Check sheet for the modelled part. Datum: model origin and axes. Units: mm. A direction names the side the tool comes from. Coordinates: 2 decimals unless noted, no trailing zeros. Order: outer loops, then holes, each group sorted by start corner. A loop starts at its lowest first (then second) coordinate and runs counter-clockwise, first axis right, second up. Notation, with made-up numbers: (-37.5, -8) -> (-33.5, -8) arc R35 ccw to (-33.5, 25) -> close; hole circle Ø5 at (16, 46.25). An arc over 180 degrees is marked (long way). Put each result on its own line as item: value. Start each with the question number.
```python
from build123d import *

# Parameters (mm, degrees)
BOSS_EXTRUDE1_DEPTH = 7
SKETCH2_R           = 7
SKETCH2_R_2         = 4
BOSS_EXTRUDE2_DEPTH = 5
SKETCH3_R           = 4
CUT_EXTRUDE1_DEPTH  = 15
BOSS_EXTRUDE3_DEPTH = 12
SKETCH5_R           = 1.5
CUT_EXTRUDE2_DEPTH  = 12


with BuildPart() as part:
    # Sketch1 → Boss-Extrude1 (new body)
    with BuildSketch(Plane.XY):
        with BuildLine():
            ThreePointArc((-12.439687438, -6.422941417), (-10.325628022, -6.417742109), (-8.410516827, -5.522407894))
            ThreePointArc((-8.410516827, -5.522407894), (-7.866397461, -6.273242641), (-7.255465658, -6.970796248))
            ThreePointArc((-7.255465658, -6.970796248), (-8.554504306, -8.638661002), (-9.029995733, -10.698559579))
            ThreePointArc((-9.029995733, -10.698559579), (-8.728857226, -10.945640755), (-8.42096127, -11.184248356))
            ThreePointArc((-8.42096127, -11.184248356), (-6.518515447, -10.262307937), (-5.181530838, -8.624704077))
            ThreePointArc((-5.181530838, -8.624704077), (-4.365521241, -9.065098264), (-3.512433539, -9.428498973))
            ThreePointArc((-3.512433539, -9.428498973), (-3.959167524, -11.494824938), (-3.493813999, -13.557037425))
            ThreePointArc((-3.493813999, -13.557037425), (-3.115293075, -13.648990771), (-2.734360446, -13.730377742))
            ThreePointArc((-2.734360446, -13.730377742), (-1.420330943, -12.07429782), (-0.926279119, -10.018771843))
            ThreePointArc((-0.926279119, -10.018771843), (0, -10.0615), (0.926279119, -10.018771843))
            ThreePointArc((0.926279119, -10.018771843), (1.420330943, -12.07429782), (2.734360446, -13.730377742))
            ThreePointArc((2.734360446, -13.730377742), (3.115293075, -13.648990771), (3.493813999, -13.557037425))
            ThreePointArc((3.493813999, -13.557037425), (3.959167524, -11.494824938), (3.512433539, -9.428498973))
            ThreePointArc((3.512433539, -9.428498973), (4.365521241, -9.065098264), (5.181530838, -8.624704077))
            ThreePointArc((5.181530838, -8.624704077), (6.518515447, -10.262307937), (8.42096127, -11.184248356))
            ThreePointArc((8.42096127, -11.184248356), (8.728857226, -10.945640755), (9.029995733, -10.698559579))
            ThreePointArc((9.029995733, -10.698559579), (8.554504306, -8.638661002), (7.255465658, -6.970796248))
            ThreePointArc((7.255465658, -6.970796248), (7.866397461, -6.273242641), (8.410516827, -5.522407894))
            ThreePointArc((8.410516827, -5.522407894), (10.325628022, -6.417742109), (12.439687438, -6.422941417))
            ThreePointArc((12.439687438, -6.422941417), (12.613564151, -6.074372348), (12.777676066, -5.7211008))
            ThreePointArc((12.777676066, -5.7211008), (11.455516597, -4.071504309), (9.561463821, -3.132441835))
            ThreePointArc((9.561463821, -3.132441835), (9.809237188, -2.238894377), (9.97369681, -1.3263311))
            ThreePointArc((9.97369681, -1.3263311), (12.087623332, -1.302063747), (13.994580946, -0.389492158))
            ThreePointArc((13.994580946, -0.389492158), (14, 0), (13.994580946, 0.389492158))
            ThreePointArc((13.994580946, 0.389492158), (12.087623332, 1.302063747), (9.97369681, 1.3263311))
            ThreePointArc((9.97369681, 1.3263311), (9.809237188, 2.238894377), (9.561463821, 3.132441835))
            ThreePointArc((9.561463821, 3.132441835), (11.455516597, 4.071504309), (12.777676066, 5.7211008))
            ThreePointArc((12.777676066, 5.7211008), (12.613564151, 6.074372348), (12.439687438, 6.422941417))
            ThreePointArc((12.439687438, 6.422941417), (10.325628022, 6.417742109), (8.410516827, 5.522407894))
            ThreePointArc((8.410516827, 5.522407894), (7.866397461, 6.273242641), (7.255465658, 6.970796248))
            ThreePointArc((7.255465658, 6.970796248), (8.554504306, 8.638661002), (9.029995733, 10.698559579))
            ThreePointArc((9.029995733, 10.698559579), (8.728857226, 10.945640755), (8.42096127, 11.184248356))
            ThreePointArc((8.42096127, 11.184248356), (6.518515447, 10.262307937), (5.181530838, 8.624704077))
            ThreePointArc((5.181530838, 8.624704077), (4.365521241, 9.065098264), (3.512433539, 9.428498973))
            ThreePointArc((3.512433539, 9.428498973), (3.959167524, 11.494824938), (3.493813999, 13.557037425))
            ThreePointArc((3.493813999, 13.557037425), (3.115293075, 13.648990771), (2.734360446, 13.730377742))
            ThreePointArc((2.734360446, 13.730377742), (1.420330943, 12.07429782), (0.926279119, 10.018771843))
            ThreePointArc((0.926279119, 10.018771843), (0, 10.0615), (-0.926279119, 10.018771843))
            ThreePointArc((-0.926279119, 10.018771843), (-1.420330943, 12.07429782), (-2.734360446, 13.730377742))
            ThreePointArc((-2.734360446, 13.730377742), (-3.115293075, 13.648990771), (-3.493813999, 13.557037425))
            ThreePointArc((-3.493813999, 13.557037425), (-3.959167524, 11.494824938), (-3.512433539, 9.428498973))
            ThreePointArc((-3.512433539, 9.428498973), (-4.365521241, 9.065098264), (-5.181530838, 8.624704077))
            ThreePointArc((-5.181530838, 8.624704077), (-6.518515447, 10.262307937), (-8.42096127, 11.184248356))
            ThreePointArc((-8.42096127, 11.184248356), (-8.728857226, 10.945640755), (-9.029995733, 10.698559579))
            ThreePointArc((-9.029995733, 10.698559579), (-8.554504306, 8.638661002), (-7.255465658, 6.970796248))
            ThreePointArc((-7.255465658, 6.970796248), (-7.866397461, 6.273242641), (-8.410516827, 5.522407894))
            ThreePointArc((-8.410516827, 5.522407894), (-10.325628022, 6.417742109), (-12.439687438, 6.422941417))
            ThreePointArc((-12.439687438, 6.422941417), (-12.613564151, 6.074372348), (-12.777676066, 5.7211008))
            ThreePointArc((-12.777676066, 5.7211008), (-11.455516597, 4.071504309), (-9.561463821, 3.132441835))
            ThreePointArc((-9.561463821, 3.132441835), (-9.809237188, 2.238894377), (-9.97369681, 1.3263311))
            ThreePointArc((-9.97369681, 1.3263311), (-12.087623332, 1.302063747), (-13.994580946, 0.389492158))
            ThreePointArc((-13.994580946, 0.389492158), (-14, 0), (-13.994580946, -0.389492158))
            ThreePointArc((-13.994580946, -0.389492158), (-12.087623332, -1.302063747), (-9.97369681, -1.3263311))
            ThreePointArc((-9.97369681, -1.3263311), (-9.809237188, -2.238894377), (-9.561463821, -3.132441835))
            ThreePointArc((-9.561463821, -3.132441835), (-11.455516597, -4.071504309), (-12.777676066, -5.7211008))
            ThreePointArc((-12.777676066, -5.7211008), (-12.613564151, -6.074372348), (-12.439687438, -6.422941417))
        make_face()
    extrude(amount=BOSS_EXTRUDE1_DEPTH)

    # Sketch2 → Boss-Extrude2 (add)
    with BuildSketch(Plane.XY.offset(7)):
        Circle(SKETCH2_R)
        Circle(SKETCH2_R_2, mode=Mode.SUBTRACT)
    extrude(amount=BOSS_EXTRUDE2_DEPTH)

    # Sketch3 → Cut-Extrude1 (cut)
    with BuildSketch(Plane.XY.offset(7)):
        Circle(SKETCH3_R)
    extrude(amount=-CUT_EXTRUDE1_DEPTH, mode=Mode.SUBTRACT)

    # Sketch4 → Boss-Extrude3 (add)
    with BuildSketch(Plane(origin=(0, 0, 0), x_dir=(-1, 0, 0), z_dir=(0, 0, -1))):
        with BuildLine():
            Line((3.841780502, 1.113877271), (0.246510723, -3.992396832))
            ThreePointArc((0.246510723, -3.992396832), (3.27063298, -2.302815648), (3.841780502, 1.113877271))
        make_face()
    extrude(amount=-BOSS_EXTRUDE3_DEPTH)

    # Sketch5 → Cut-Extrude2 (cut)
    with BuildSketch(Plane(origin=(-10.220728062, -7.196298901, 0), x_dir=(0, 0, -1), z_dir=(0.817658245, 0.575703912, 0))):
        with Locations((-9.5, 0)):
            Circle(SKETCH5_R)
    extrude(amount=CUT_EXTRUDE2_DEPTH, mode=Mode.SUBTRACT)


solid = part.part
```
1) Scan lines: line 1 along Y through (x, z) = (-10.75, 2.5); line 2 along Y through (x, z) = (0, 5.25); line 3 along X through (y, z) = (-9.25, 4.5). Record each from-to range of solid material in increasing order. Write a range as [from, to].
2) Mould release check, pull along Y, two halves, no side actions. Record for faces 1 (the flat face through (-6.4, 3.2, 7)), 2 (the cylindrical face through (-9.806, 2.252, 3.451)), 3 (the cylindrical face through (6.495, -10.244, 3.451)), 4 (the cylindrical face through (-3.96, -11.46, 3.45)): +Y half, -Y half, draft (parallel to the pull), parting line (faces both ways), or undercut.
3) Sectioned sample at B-B (z = 9). Record the boundary of the cut face in (x, y).
4) Sectioned sample at A-A (x = -7.75). Record the boundary of the cut face in (y, z), plus the area to 3 significant figures.
5) Gauge pin test, flat ends, axial feed: pin 1 (6.5 mm diameter, centred on x = 0, y = 0, fed in from +Z); pin 2 (1 mm diameter, centred on x = 10, z = 3.5, fed in from +Y); pin 3 (1.5 mm diameter, centred on y = -3, z = 7, fed in from +X); pin 4 (2 mm diameter, centred on y = -6, z = 4.5, fed in from +X). Record the tip position at first contact, or that the pin passes through.
6) Access from +Z, -Z, +X, -X, +Y, -Y to the whole of each face (thin tool, end or side, straight path). Record for faces 5 (the cylindrical face through (3.763, 5.902, 9.465)), 6 (the cylindrical face through (7.86, -6.28, 3.45)), 7 (the cylindrical face through (-1.433, -12.101, 3.451)), 8 (the cylindrical face through (-8.54, -8.61, 3.45)), 9 (the flat face through (-3, -3, 0)).
Entries:
1. line 1: y = [-6.49, -3.6], [-1.42, 1.42], [3.6, 6.49]
1. line 2: y = [-10.06, -4], [4, 10.06]
1. line 3: x = [-8.8, -5.56], [-3.96, 3.96], [5.56, 8.8]
2. face 1: draft
2. face 2: undercut
2. face 3: -Y half
2. face 4: undercut
3. outline: (-6.42, -2.79) -> (-2.86, -0.28) -> (-3.84, 1.11) arc R4 cw (long way) to (-0.25, -3.99) -> (-1.23, -2.6) -> (-4.79, -5.1) arc R7 ccw (long way) to start
4. outline: (-10.97, 0) -> (-7.44, 0) -> (-7.44, 7) -> (-10.97, 7) -> close; (-6.42, 0) -> (6.42, 0) -> (6.42, 7) -> (-6.42, 7) -> close; (7.44, 0) -> (10.97, 0) -> (10.97, 7) -> (7.44, 7) -> close
4. area: 139 mm2
5. pin 1: stops at z = 12
5. pin 2: stops at y = 6.45
5. pin 3: stops at x = 11.01
5. pin 4: stops at x = 12.78
6. face 5: +Z
6. face 6: +Z, -Z
6. face 7: +Z, -Z, -Y
6. face 8: +Z, -Z, -X
6. face 9: -Z, +X, -X, +Y, -Y
